Geometry check sheet. Reference: the model listing, model coordinates, mm. Round coordinates to 2 decimals unless told otherwise and drop trailing zeros. Loops run counter-clockwise (first coordinate to the right, second up) from the corner with the lowest first, then second, coordinate; pieces in that order, holes last. Notation, with made-up numbers: (-32, -24) -> (18, -24) arc R16 ccw to (18, -10) -> close; hole circle Ø11 at (42.25, 71). An arc over 180 degrees is marked (long way). Use a Markdown table: item, result. Add a question column.
Q1. Material ranges on L1, parallel to Z at x = -54.5, y = -19; L2, parallel to Y at x = -83, z = 63; L3, parallel to X at y = -64, z = 119.5, recorded low to high.
Q2. Gauge pin test, flat ends, axial feed: P1, Ø12, axis at y = -3, z = 24, coming from the +X side; P2, Ø2, axis at y = -80, z = 38.5, coming from the +X side; P3, Ø1, axis at x = -63.5, y = -51.5, coming from the +Z side. Record the tip position at first contact, or that the pin passes through.
Q3. Sectioned sample at A-A, the plane z = 43. Enter the section's corners in (x, y).
Q4. Sectioned sample at B-B, the plane z = 107. Enter the section's corners in (x, y), then the cut area to 3 significant figures.
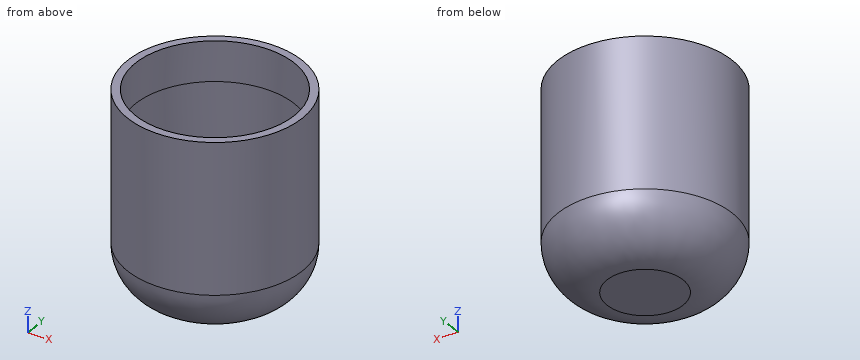
```python
from build123d import *

# Parameters (mm, degrees)
F0_R     = 55
F1_DEPTH = 100
F2_R     = 31
F3_R     = 50
F4_DEPTH = 70
F5_DEPTH = 25


with BuildPart() as f1:
    # F0 (on Top) → F1 (new body)
    with BuildSketch(Plane.XY):
        with Locations((-64.8039355874, -38.4441465139)):
            Circle(F0_R)
    extrude(amount=F1_DEPTH)

    # F2
    f2_edges = [f1.edges().sort_by_distance(p)[0] for p in [
        (-119.803936, -38.444147, 0),
    ]]
    fillet(f2_edges, radius=F2_R)

    # F3 (on face) → F4 (cut)
    with BuildSketch(Plane.XY.offset(100)):
        with Locations((-64.8039355874, -38.4441465139)):
            Circle(F3_R)
    extrude(amount=-F4_DEPTH, mode=Mode.SUBTRACT)

    # F5 (add): faces of the model
    f5_faces = [f1.faces().sort_by_distance(p)[0] for p in [
        (-118.2483006688, -38.4441465139, 100),
        (-64.8039355874, -38.4441465139, 30),
    ]]
    extrude(f5_faces, amount=F5_DEPTH)


solid = f1.part
```
Values:
| question | item | result |
|---|---|---|
| 1 | L1 | 0 to 55 |
| 1 | L2 | -90.35 to -85.02, 8.13 to 13.46 |
| 1 | L3 | -113.51 to -107.78, -21.83 to -16.1 |
| 2 | P1 | x = -19.05 |
| 2 | P2 | x = -27.65 |
| 2 | P3 | z = 55 |
| 3 | outline | circle Ø110 at (-64.8, -38.44) |
| 4 | outline | circle Ø110 at (-64.8, -38.44); hole circle Ø100 at (-64.8, -38.44) |
| 4 | area | 1,650 mm^2 |
